Model file for the job. Use its own axes, mm. A direction names the side the tool comes from. Coordinates: 2 decimals unless noted, no trailing zeros. Loops run counter-clockwise (first coordinate to the right, second up) from the corner with the lowest first, then second, coordinate; pieces in that order, holes last.
from build123d import *

# Parameters (mm, degrees)
HOLE1_D           = 9.73836
HOLE1_DEPTH       = 28.062477616
HOLE1_CSINK_D     = 11.1125
HOLE1_CSINK_ANGLE = 90
HOLE1_TIP         = 2.811222384


with BuildPart() as part:
    # Sketch1 → Revolve1 (revolve)
    with BuildSketch(Plane.XY):
        Polygon((-22.225, 0), (-22.225, 8.001), (119.9642, 8.001), (119.9642, 25.4508), (148.4376, 25.4508), (148.4376, 0), align=None)
    revolve(axis=Axis((148.4376, 0, 0), (-1, 0, 0)))

    # Hole1
    with Locations(Plane.ZY.offset(22.225)):
        with Locations((0, 0)):
            CounterSinkHole(HOLE1_D / 2, HOLE1_CSINK_D / 2, depth=HOLE1_DEPTH, counter_sink_angle=HOLE1_CSINK_ANGLE)
            with Locations((0, 0, -(HOLE1_DEPTH + HOLE1_TIP / 2))):  # 120° drill point
                Cone(0, HOLE1_D / 2, HOLE1_TIP, mode=Mode.SUBTRACT)


solid = part.part
Q1. Flat gauge pins, fed straight in: P1, Ø12, axis at x = 67.5, y = -14.5, coming from the -Z side; P2, Ø2, axis at y = 17, z = -20, coming from the -X side; P3, Ø6, axis at y = 0, z = 0, coming from the -X side; P4, Ø8, axis at x = -3, y = -2, coming from the +Z side. Where does each tip first touch, or does it go through?
Answers:
P1: passes through
P2: stops at x = 119.96
P3: stops at x = 6.92
P4: stops at z = 8
Q2. Slice it at C-C (z = 14). List the corners of the cut face in (x, y), and give its area (3 significant figures).
Answers:
outline: (119.96, -21.25) - (148.44, -21.25) - (148.44, 21.25) - (119.96, 21.25) - close
area: 1,210 mm2
Q3. Mould opens along Z. For faces 3 (the flat face through (-22.225, 1.9, -5.4)), 4 (the conical face through (8.16, -0.83, -0.18)), 5 (the cylindrical face through (134.4, -3.313, -25.234)), 6 (the cylindrical face through (-7.659, -4.753, 1.056)) say: +Z half, -Z half, draft (parallel to the pull), parting line (faces both ways), or undercut.
Answers:
face 3: draft
face 4: undercut
face 5: parting line
face 6: undercut
Q4. Which spindle directions (+Z, -Z, +X, -X, +Y, -Y) get a long thin tool onto all of the face, cutting with end or side? Do faces 1 (the flat face through (119.964, 6, -6)), 2 (the flat face through (148.438, 0, 0)). Say none if no direction does.
Answers:
face 1: -X
face 2: +Z, -Z, +X, +Y, -Y
Q5. Slice it at B-B (y = 16). List the corners of the cut face in (x, z), and give its area (3 significant figures).
Answers:
outline: (119.96, -19.79) - (148.44, -19.79) - (148.44, 19.79) - (119.96, 19.79) - close
area: 1,130 mm2
Q6. Slice it at D-D (x = 124.5). List the corners of the cut face in (y, z).
Answers:
outline: circle Ø50.9 at (0, 0)
Q7. Slice it at A-A (x = 99.5). List the corners of the cut face in (y, z), and give its area (3 significant figures).
Answers:
outline: circle Ø16 at (0, 0)
area: 201 mm2
Q8. Drill centre lines: line 1 (Y direction, x = -14.25, z = 0); line 2 (X direction, y = -3.5, z = 16). Where is each one in solid material? Low to high.
Answers:
line 1: y = -8 to -4.87, 4.87 to 8
line 2: x = 119.96 to 148.44
